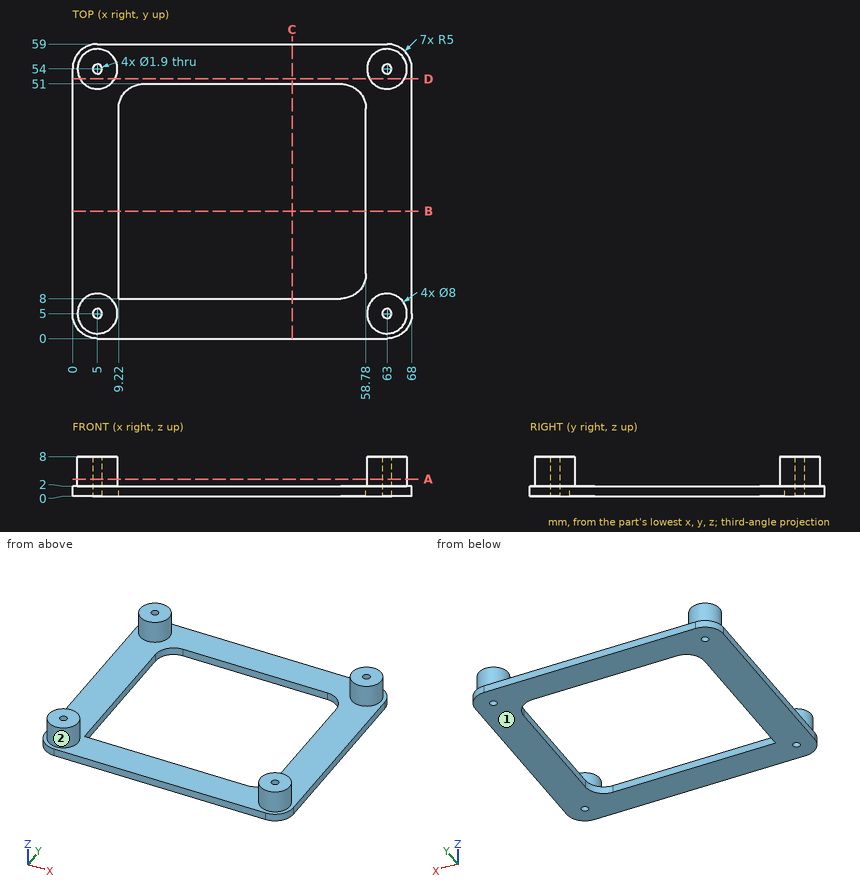
Verification items for this drawing (mm, ordinates from the low corner). Round coordinates to 2 decimals unless told otherwise and drop trailing zeros. Write each loop counter-clockwise with the first axis right and the second up, starting at its lowest first coordinate (ties: lowest second). Pieces come first, ordered by that corner, then holes. Notation, with made-up numbers: (87.5, 20.5) - (103.5, 20.5) arc R3 ccw to (103.5, 25.5) - close; hole circle Ø7 at (3, 41.25). An arc over 180 degrees is marked (long way). Answer as a JSON object with one key per item and string values. Group by question number.
Q1. Mould release check, pull along Y, two halves, no side actions. Record for the marked faces 1 and 2: released by +Y, released by -Y, zero draft, split by the parting line, or undercut.
Q2. Section check D-D, the plane y = 52. Enter the section's corners in (x, z), plus the area to 3 significant figures.
Q3. Go/stop test with a flat-tipped pin: pin 1 Ø2 at (x, z) = (58.5, 4.5) entering from -Y (1 decimal). Record where the tip stops, or that it passes through.
Q4. Thickness scan on line 1 (Y direction, x = 63, z = 5); line 2 (X direction, y = 54, z = 4); line 3 (X direction, y = 45.5, z = 1.5). Record the ranges inside material, lowest first.
Q5. Section check C-C, the plane x = 44. Enter the section's corners in (y, z).
Q6. Section check A-A, the plane z = 3.5. Enter the section's corners in (x, y).
Q7. Section check B-B, the plane y = 25.5. Enter the section's corners in (x, z).
Found:
{
 "1": {"face 1": "zero draft", "face 2": "undercut"},
 "2": {"outline": "(0, 0) - (68, 0) - (68, 2) - (66.46, 2) - (66.46, 8) - (59.54, 8) - (59.54, 2) - (8.46, 2) - (8.46, 8) - (1.54, 8) - (1.54, 2) - (0, 2) - close", "area": "219 mm^2"},
 "3": {"pin 1": "stops at y = 3.1"},
 "4": {"line 1": "y = 1 to 4.05, 5.95 to 9, 50 to 53.05, 54.95 to 58", "line 2": "x = 1 to 4.05, 5.95 to 9, 59 to 62.05, 63.95 to 67", "line 3": "x = 0 to 9.22, 58.78 to 68"},
 "5": {"outline": "(0, 0) - (8, 0) - (8, 2) - (0, 2) - close; (51, 0) - (59, 0) - (59, 2) - (51, 2) - close"},
 "6": {"outline": "circle Ø8 at (5, 5); circle Ø8 at (5, 54); circle Ø8 at (63, 5); circle Ø8 at (63, 54); hole circle Ø1.9 at (5, 5); hole circle Ø1.9 at (5, 54); hole circle Ø1.9 at (63, 5); hole circle Ø1.9 at (63, 54)"},
 "7": {"outline": "(0, 0) - (9.22, 0) - (9.22, 2) - (0, 2) - close; (58.78, 0) - (68, 0) - (68, 2) - (58.78, 2) - close"}
}
